Check sheet for the modelled part. Datum: model origin and axes. Units: mm. A direction names the side the tool comes from. Give positions to 0.01 mm unless a question says otherwise; leave off trailing zeros. Order: outer loops, then holes, each group sorted by start corner. A loop starts at its lowest first (then second) coordinate and runs counter-clockwise, first axis right, second up. Notation, with made-up numbers: M -15.75,50.25 L 33.25,50.25 A26 cw 33.25,75.25 Z; hole C -28,50 d1. An arc over 180 degrees is marked long. Return JSON: item names as keys, results as strings. Group by question number.
from build123d import *

# Parameters (mm, degrees)
SKETCH1_R           = 1.7
BOSS_EXTRUDE1_DEPTH = 5
SKETCH2_R           = 4.75
BOSS_EXTRUDE2_DEPTH = 7
FILLET1_R           = 1.5


with BuildPart() as part:
    # Sketch1 → Boss-Extrude1 (new body)
    with BuildSketch(Plane(origin=(0, 0, 0), x_dir=(1, 0, 0), z_dir=(0, 1, 0))):
        with BuildLine():
            Line((-26.16880337, -11.602959843), (-15.107142779, 0.343633596))
            ThreePointArc((-15.107142779, 0.343633596), (-13.981683241, 5.160195913), (-17.548068062, 8.58756094))
            Line((-17.548068062, 8.58756094), (-23.727878087, 10.153112813))
            ThreePointArc((-23.727878087, 10.153112813), (-27.461574142, 15.618693812), (-22.5, 20))
            Line((-22.5, 20), (22.5, 20))
            ThreePointArc((22.5, 20), (27.461574142, 15.618693812), (23.727878087, 10.153112813))
            Line((23.727878087, 10.153112813), (17.548068062, 8.58756094))
            ThreePointArc((17.548068062, 8.58756094), (13.981683241, 5.160195913), (15.107142779, 0.343633596))
            Line((15.107142779, 0.343633596), (26.16880337, -11.602959843))
            ThreePointArc((26.16880337, -11.602959843), (25.897040157, -18.66880337), (18.83119663, -18.397040157))
            Line((18.83119663, -18.397040157), (3.66880337, -2.021655437))
            ThreePointArc((3.66880337, -2.021655437), (0, -0.418695594), (-3.66880337, -2.021655437))
            Line((-3.66880337, -2.021655437), (-18.83119663, -18.397040157))
            ThreePointArc((-18.83119663, -18.397040157), (-25.897040157, -18.66880337), (-26.16880337, -11.602959843))
        make_face()
        with Locations(Location((22.5, 15, 0), (0, 0, 270))):
            Circle(SKETCH1_R, mode=Mode.SUBTRACT)
        with Locations(Location((22.5, -15, 0), (0, 0, 270))):
            Circle(SKETCH1_R, mode=Mode.SUBTRACT)
        with Locations(Location((-22.5, 15, 0), (0, 0, 270))):
            Circle(SKETCH1_R, mode=Mode.SUBTRACT)
        with Locations(Location((-22.5, -15, 0), (0, 0, 270))):
            Circle(SKETCH1_R, mode=Mode.SUBTRACT)
    extrude(amount=BOSS_EXTRUDE1_DEPTH)

    # Sketch2 → Boss-Extrude2 (add)
    with BuildSketch(Plane(origin=(0, 5, 0), x_dir=(1, 0, 0), z_dir=(0, 1, 0))):
        with Locations(Location((0, 9.3, 0), (0, 0, 270))):
            Circle(SKETCH2_R)
    extrude(amount=BOSS_EXTRUDE2_DEPTH)

    # Fillet1
    fillet1_edges = [part.edges().sort_by_distance(p)[0] for p in [
        (-20.637973075, 0, 5.629663123),
        (-13.981683241, 0, -5.160195913),
        (-20.637973075, 0, -9.370336877),
        (-27.461574142, 0, -15.618693812),
        (0, 0, -20),
        (27.461574142, 0, -15.618693812),
        (20.637973075, 0, -9.370336877),
        (13.981683241, 0, -5.160195913),
        (20.637973075, 0, 5.629663123),
        (25.897040157, 0, 18.66880337),
        (11.25, 0, 10.209347797),
        (0, 0, 0.418695594),
        (-11.25, 0, 10.209347797),
        (-25.897040157, 0, 18.66880337),
    ]]
    fillet(fillet1_edges, radius=FILLET1_R)


solid = part.part
1) Depth check by flat-ended pin: P1, Ø4, axis at x = -22.5, z = -15, coming from the -Y side; P2, Ø3, axis at x = 6, z = 6.5, coming from the +Y side. Enter the tip coordinate at first touch or a pass-through.
2) Tool access check on faces 1 (the face through (-11.14, 3.23, 10.09)), 2 (the face through (-20.58, 0.45, -9.8)), 3 (the face through (-20.59, 3.23, -9.36)). Record the directions out of +Z, -Z, +X, -X, +Y, -Y that give a thin tool (end or side, any length) a straight path to the whole face; none if there is none.
3) Release check for a two-part mould opening along X. For faces 4 (the face through (-25.82, 3.23, 18.74)), 5 (the face through (-27.473, 3.226, -15.518)), 6 (the face through (1.43, 8.45, -4.77)), 7 (the face through (20.49, 0.451, -9.774)) record: released by +X, released by -X, zero draft, split by the parting line, or undercut.
4) Sectioned sample at D-D on y = 10.25. Record the boundary of the cut face in (x, z).
5) Material ranges on line 1 along X through (y, z) = (2.7, -15); line 2 along X through (y, z) = (1.05, 15); line 3 along X through (y, z) = (3.35, 15), recorded low to high.
6) Sectioned sample at A-A on y = 2.5. Record the boundary of the cut face in (x, z).
7) Sectioned sample at C-C on z = -15. State how many separate pieces and enclosed holes the cut face has, then the cut area to 3 significant figures.
8) Sectioned sample at B-B on x = 0. Record the boundary of the cut face in (y, z).
Reply:
{
 "1": {"P1": "y = 0", "P2": "y = 5"},
 "2": {"face 1": "+Z, +Y, -Y", "face 2": "-X, -Y", "face 3": "-X, +Y, -Y"},
 "3": {"face 4": "undercut", "face 5": "released by -X", "face 6": "split by the parting line", "face 7": "released by +X"},
 "4": {"outline": "C 0,-9.3 d9.5"},
 "5": {"line 1": "-27.5 to -24.2, -20.8 to 20.8, 24.2 to 27.5", "line 2": "-27.43 to -24.2, -20.8 to -15.78, 15.78 to 20.8, 24.2 to 27.43", "line 3": "-27.5 to -24.2, -20.8 to -15.69, 15.69 to 20.8, 24.2 to 27.5"},
 "6": {"outline": "M -26.17,11.6 L -15.11,-0.34 A5 cw -17.55,-8.59 L -23.73,-10.15 A5 ccw -22.5,-20 L 22.5,-20 A5 ccw 23.73,-10.15 L 17.55,-8.59 A5 cw 15.11,-0.34 L 26.17,11.6 A5 ccw 18.83,18.4 L 3.67,2.02 A5 cw -3.67,2.02 L -18.83,18.4 A5 ccw Z; hole C -22.5,-15 d3.4; hole C -22.5,15 d3.4; hole C 22.5,-15 d3.4; hole C 22.5,15 d3.4"},
 "7": {"separate pieces": "3", "enclosed holes": "0", "area": "240 mm^2"},
 "8": {"outline": "M 0,-18.5 A1.5 ccw 1.5,-20 L 5,-20 L 5,-14.05 L 12,-14.05 L 12,-4.55 L 5,-4.55 L 5,0.42 L 1.5,0.42 A1.5 ccw 0,-1.08 Z"}
}
